Design review of the part built by this model. Coordinates are the model's own, in mm. Face numbers are marked on the shaded views. A direction names the side the tool comes from. Coordinates: 2 decimals unless noted, no trailing zeros. Loops run counter-clockwise (first coordinate to the right, second up) from the corner with the lowest first, then second, coordinate; pieces in that order, holes last. Notation, with made-up numbers: (53.5, 61) - (76.5, 61) arc R19 cw to (76.5, 87) - close; hole circle Ø11 at (-8, 1.25). An arc over 180 degrees is marked (long way). Use one line per item in the form item = value. Start each with the question number.
(1) Add section A-A (x = 0). State the section outline as (y, z) points, plus the area to 3 significant figures.
(2) Clearance check with flat-ended pins moving along their axes: pin 1 Ø2 at (y, z) = (1, 10) entering from -X; pin 2 Ø3 at (x, y) = (-4.5, -4) entering from +Z; pin 3 Ø5 at (x, y) = (1.5, -1) entering from +Z; pin 4 Ø4 at (x, z) = (0, 0) entering from -Y. State where each tip first meets the part, or that it passes through.
(3) For L1, parallel to Y at x = -9, z = 7.25; L2, parallel to X at y = -2, z = -10; L3, parallel to X at y = 2, z = -7.25, list the stretches that pass through material, from the lowest coordinate up.
(4) The part is to be moulded in two halves that separate along Z. For the marked faces 1, 2 and 3, say which applies: pulls with the +Z half, pulls with the -Z half, needs draft (parallel to the pull), parting line crosses it, or undercut.
(5) Tool access review of the marked faces 4, 5 and 6: name each direction out of +Z, -Z, +X, -X, +Y, -Y from which nothing blocks a thin tool from reaching the whole face with its end or side.
```python
from build123d import *

# Parameters (mm, degrees)
SKETCH2_W          = 1.5
SKETCH2_H          = 10
CUT_EXTRUDE1_DEPTH = 2
CIRPATTERN1_COUNT  = 21


with BuildPart() as part:
    # Sketch1 → Revolve1 (revolve)
    with BuildSketch(Plane.XY, mode=Mode.PRIVATE) as revolve1_sk:
        Polygon((2.5, -5.930921053), (4.177631579, -5.930921053), (12, -5.930921053), (12, -4.930921053), (11, -4.930921053), (11, 5.069078947), (12, 5.069078947), (12, 6.069078947), (4.177631579, 6.069078947), (2.5, 6.069078947), align=None)
    revolve(revolve1_sk.sketch.rotate(Axis((0, 0, 0), (0, 1, 0)), 90), axis=Axis((0, 0, 0), (0, 1, 0)))  # turned: the seam where the file's is

    # Sketch2 → Cut-Extrude1 (cut)
    with BuildSketch(Plane.XY.offset(11)):
        with Locations((0, 0.069078947)):
            Rectangle(SKETCH2_W, SKETCH2_H)
    cut_extrude1 = extrude(amount=-CUT_EXTRUDE1_DEPTH, mode=Mode.SUBTRACT)

    # CirPattern1: Cut-Extrude1 ×21 about axis
    cirpattern1_axis = Axis((0, 0, 0), (0, 1, 0))
    for i in range(1, CIRPATTERN1_COUNT):
        add(cut_extrude1.rotate(cirpattern1_axis, i * 360 / CIRPATTERN1_COUNT), mode=Mode.SUBTRACT)


solid = part.part
```
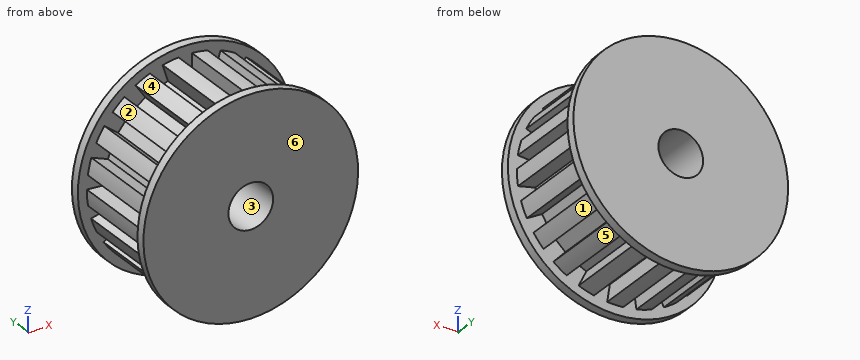
Computed values:
q1.outline = (-5.93, -12) - (-4.93, -12) - (-4.93, -11) - (5.07, -11) - (5.07, -12) - (6.07, -12) - (6.07, -2.5) - (-5.93, -2.5) - close; (-5.93, 2.5) - (6.07, 2.5) - (6.07, 12) - (5.07, 12) - (5.07, 9) - (-4.93, 9) - (-4.93, 12) - (-5.93, 12) - close
q1.area = 188 mm^2
q2.pin_1 = -5.56
q2.pin_2 = 11.53
q2.pin_3 = 10.97
q2.pin_4 = through
q3.L1 = -5.93 to -4.93, 5.07 to 6.07
q3.L2 = -3.98 to -2.27, -0.75 to 0.75, 2.27 to 3.98
q3.L3 = -8.27 to -7.75, -5.7 to 5.7, 7.75 to 8.27
q4.face_1 = pulls with the -Z half
q4.face_2 = pulls with the +Z half
q4.face_3 = undercut
q5.face_4 = +Z, -X
q5.face_5 = -Z, +X
q5.face_6 = +Z, -Z, +X, -X, -Y
